Autodesk Inventor part; units mm, degrees
ref_plane "YZ Plane" through (0, 0, 0) normal (1, 0, 0) x (0, 1, 0)
ref_plane "XZ Plane" through (0, 0, 0) normal (0, 1, 0) x (-1, 0, 0)
ref_plane "XY Plane" through (0, 0, 0) normal (0, 0, 1) x (1, 0, 0)
sketch "Sketch1" plane through (0, 0, 0) normal (0, 0, 1) x (1, 0, 0)
  line L0 (0, 0) -> (0, 40)
  line L1 (0, 0) -> (61, 0)
  line L2 (61, 0) -> (61, 5)
  line L3 (61, 5) -> (7, 5)
  arc A0 (7, 40) -> (0, 40) centre (3.5, 40) ccw
  line L4 (7, 40) -> (7, 5)
  circle A1 centre (3.5, 40) radius 2.5
  dimension "d0" = 40
  dimension "d2" = 5
  dimension "d6" = 3.5
  dimension "d7" = 5
  dimension "d8" = 7
  dimension "d9" = 54
  dimension "d46" = 61
extrude "Extrusion1" add sketch "Sketch1" along normal blind 20
sketch "Sketch2" plane through (7, 5, 0) normal (0, 1, 0) x (1, 0, 0)
  circle A0 centre (6.5, -10) radius 1.5
  line L0 (0, 0) -> (0, -20)
  circle A1 centre (23, -10) radius 10
  line L1 (0, 0) -> (54, 0)
  circle A2 centre (52, -10) radius 2
  line L2 (54, 0) -> (54, -20)
  line L3 (-1, 0) -> (-1, -20)
  line L4 (-6, 0) -> (-6, -20)
  line L5 (-7, -10) -> (-7, -6.6929)
  point P0 (-7, 0)
  dimension "d12" = 3
  dimension "d13" = 6.5
  dimension "d14" = 20
  dimension "d16" = 23
  dimension "d19" = 10
  dimension "d20" = 4
  dimension "d21" = 10
  dimension "d22" = 17
  dimension "d47" = 31
  dimension "d48" = 59
  dimension "d49" = 30
  dimension "d50" = 13.5
extrude "Extrusion2" add sketch "Sketch2" along normal blind 20
sketch "Sketch4" plane through (0, 0, 20) normal (0, 0, 1) x (1, 0, 0)
  line L0 (15, 25) -> (12, 25)
  line L1 (12, 25) -> (15, 25)
  line L2 (15, 5) -> (15, 25)
  line L3 (15, 25) -> (15, 15)
  line L4 (15, 15) -> (12, 15)
  line L5 (12, 5) -> (12, 25)
  point P0 (0, 0)
  dimension "d25" = 10
extrude "Extrusion3" cut sketch "Sketch4" against normal blind 20
fillet "Fillet1" radius 1 1 edges at (12, 15, 10)
fillet "Fillet2" radius 1 1 edges at (57, 25, 10)
sketch "Sketch5" plane through (30, 25, 10) normal (0, 1, 0) x (1, 0, 0)
  circle A0 centre (0, 0) radius 8
  point P0 (-30, 10)
  dimension "d30" = 16
extrude "Extrusion4" cut sketch "Sketch5" against normal blind 30
sketch "Sketch6" plane through (7, 5, 0) normal (1, 0, 0) x (0, 0, -1)
  point P0 (0, -5)
sketch "Sketch7" plane through (7, 5, 0) normal (1, 0, 0) x (0, 0, -1)
  line L0 (-10, 41.0364) -> (-10, 39.6436)
  line L1 (0, 38.5) -> (-20, 38.5)
  line L2 (-2.5, 38.5) -> (-2.5, 24.5)
  line L3 (-17.5, 38.5) -> (-17.5, 24.5)
  line L4 (-17.5, 38.5) -> (-2.5, 38.5)
  line L5 (0, 32.5) -> (-20, 32.5)
  line L6 (-17.5, 24.5) -> (-2.5, 24.5)
  point P0 (0, -5)
  dimension "d12" = 3
  dimension "d40" = 14
  dimension "d41" = 14
  dimension "d42" = 15
extrude "Extrusion5" cut sketch "Sketch7" against normal blind 14
sketch "Sketch8" plane through (30, 5, 0) normal (0, 1, 0) x (1, 0, 0)
  point P0 (-30, 0)
fillet "Fillet4" radius 3.5 2 edges at (7, 29.5, 10) (0, 29.5, 10)
equation "\"d19\" = 0.5 * d14"
equation "\"d21\" = d19"
equation "\"d40\" = d41"
properties part number "ValveBaseMk2.1"
Here's how the part is built. I have some questions about the finished solid (model axes, mm). A direction names the side the tool comes from. Coordinates: 2 decimals unless noted, no trailing zeros. Write each loop counter-clockwise with the first axis right and the second up, starting at its lowest first coordinate (ties: lowest second). Pieces come first, ordered by that corner, then holes.
Item 1: I want a section at A-A on y = 21. Write out the boundary of the cut face in (x, z), and give its area (3 significant figures).
Item 2: If I drill on line 1 (Z direction, x = 30, y = 15); line 2 (X direction, y = 10, z = 10); line 3 (Y direction, x = 3.5, z = 1.65), over which ranges is the centre line in solid material (lowest first)?
Item 3: Will these pins go through, and if not, where does the flat tip stop? pin 1 (6 mm diameter, centred on x = 18, z = 9.5, fed in from +Y); pin 2 (0.5 mm diameter, centred on x = 13.5, z = 10, fed in from +Y).
Item 4: If we mould it in two halves opening along X, with no side actions, what happens to faces 5 (the cylindrical face through (2.96, 42.44, 18.73)), 6 (the cylindrical face through (3.4, 43.5, 18.7)), 7 (the flat face through (0, 15, 10))? For each: +X half, -X half, draft (parallel to the pull), parting line (faces both ways), or undercut.
Item 5: On a 3-axis mill with a long thin cutter (end or side, diameter ignored), from which of +Z, -Z, +X, -X, +Y, -Y can I reach the whole of each face in a straight line? I mean faces 1 (the cylindrical face through (12.3, 9.4, 9.1)), 2 (the cylindrical face through (1.05, 28.5, 10.1)), 3 (the flat face through (7, 19, 10)), 4 (the flat face through (59, 25, 10)). Say none if no direction works.
Item 6: I want a section at D-D on x = 31. Write out the boundary of the cut face in (y, z).
Item 7: I want a section at B-B on y = 10. Write out the boundary of the cut face in (x, z).
Item 8: I want a section at C-C on x = 5. Write out the boundary of the cut face in (y, z), and give its area (3 significant figures).
Findings below:
1. outline: (0, 0) - (7, 0) - (7, 20) - (0, 20) - close; circle Ø20 at (30, 10); circle Ø4 at (59, 10); hole circle Ø16 at (30, 10)
1. area: 266 mm2
2. line 1: z = 0 to 2, 18 to 20
2. line 2: x = 0 to 7, 12 to 15, 20 to 22, 38 to 40, 57 to 61
2. line 3: y = 0 to 37.5, 42.5 to 43.5
3. pin 1: stops at y = 25
3. pin 2: stops at y = 15
4. face 5: undercut
4. face 6: parting line
4. face 7: -X half
5. face 1: +Y
5. face 2: -X, +Y
5. face 3: +Z, -Z, +Y
5. face 4: +Z, -Z, +X, +Y
6. outline: (0, 0) - (5, 0) - (5, 0.05) - (25, 0.05) - (25, 2.06) - (0, 2.06) - close; (0, 17.94) - (25, 17.94) - (25, 19.95) - (5, 19.95) - (5, 20) - (0, 20) - close
7. outline: (0, 0) - (7, 0) - (7, 20) - (0, 20) - close; circle Ø3 at (13.5, 10); circle Ø20 at (30, 10); circle Ø4 at (59, 10); hole circle Ø16 at (30, 10)
8. outline: (0, 0) - (38, 0) - (38, 2.5) - (29.16, 2.5) - (29.16, 17.5) - (38, 17.5) - (38, 20) - (0, 20) - close; (42, 0) - (43.16, 0) - (43.16, 2.5) - (42, 2.5) - close; (42, 17.5) - (43.16, 17.5) - (43.16, 20) - (42, 20) - close
8. area: 633 mm2
